Part print with two shaded views. Sizes in mm from the minimum x, y, z corner. Round coordinates to 2 decimals unless told otherwise and drop trailing zeros. Loops run counter-clockwise (first coordinate to the right, second up) from the corner with the lowest first, then second, coordinate; pieces in that order, holes last.
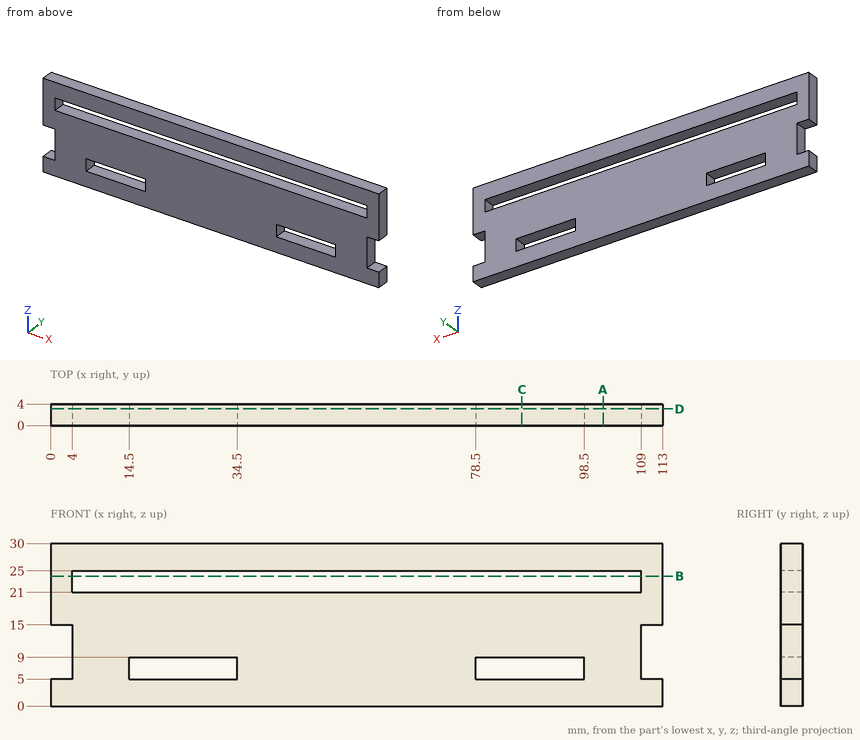
Item 1: Flat gauge pins, fed straight in: P1, Ø8, axis at x = 95, z = 8.5, coming from the +Y side; P2, Ø1, axis at y = 2.5, z = 14, coming from the +X side; P3, Ø1.2, axis at y = 2.5, z = 8.5, coming from the -X side. Where does each tip first touch, or does it go through?
Verdict:
P1: stops at y = 4
P2: stops at x = 109
P3: stops at x = 4
Item 2: Cut at A-A (x = 102). List the corners of the cut face in (y, z), plus the area to 3 significant figures.
Verdict:
outline: (0, 0) - (4, 0) - (4, 21) - (0, 21) - close; (0, 25) - (4, 25) - (4, 30) - (0, 30) - close
area: 104 mm2
Item 3: Cut at D-D (y = 3.1). List the corners of the cut face in (x, z).
Verdict:
outline: (0, 0) - (113, 0) - (113, 5) - (109, 5) - (109, 15) - (113, 15) - (113, 30) - (0, 30) - (0, 15) - (4, 15) - (4, 5) - (0, 5) - close; hole (4, 21) - (109, 21) - (109, 25) - (4, 25) - close; hole (14.5, 5) - (34.5, 5) - (34.5, 9) - (14.5, 9) - close; hole (78.5, 5) - (98.5, 5) - (98.5, 9) - (78.5, 9) - close
Item 4: Wall check: L1, parallel to Z at x = 25.5, y = 0.2; L2, parallel to Z at x = 45, y = 2.45; L3, parallel to X at y = 1.4, z = 22.5. Give the ranges that are in metal, low to high.
Verdict:
L1: z = 0 to 5, 9 to 21, 25 to 30
L2: z = 0 to 21, 25 to 30
L3: x = 0 to 4, 109 to 113
Item 5: Cut at C-C (x = 87). List the corners of the cut face in (y, z).
Verdict:
outline: (0, 0) - (4, 0) - (4, 5) - (0, 5) - close; (0, 9) - (4, 9) - (4, 21) - (0, 21) - close; (0, 25) - (4, 25) - (4, 30) - (0, 30) - close
Item 6: Cut at B-B (z = 24). List the corners of the cut face in (x, y).
Verdict:
outline: (0, 0) - (4, 0) - (4, 4) - (0, 4) - close; (109, 0) - (113, 0) - (113, 4) - (109, 4) - close
